Check sheet for the modelled part. Datum: model origin and axes. Units: mm. A direction names the side the tool comes from. Coordinates: 2 decimals unless noted, no trailing zeros. Loops run counter-clockwise (first coordinate to the right, second up) from the corner with the lowest first, then second, coordinate; pieces in that order, holes last.
```python
from build123d import *

# Parameters (mm, degrees)
SKETCH1_W           = 88.9
SKETCH1_H           = 91.44
BOSS_EXTRUDE1_DEPTH = 44.45
SKETCH2_W           = 8.382
SKETCH2_H           = 20.32
CUT_EXTRUDE1_DEPTH  = 25.4
BOSS_EXTRUDE2_DEPTH = 44.45
SKETCH4_R           = 1.6764
CUT_EXTRUDE4_DEPTH  = 22.098
SKETCH5_R           = 2.9464
CUT_EXTRUDE6_DEPTH  = 43.434
SKETCH7_W           = 12.552336234
SKETCH7_H           = 7.366
CUT_EXTRUDE7_DEPTH  = 22.098


with BuildPart() as part:
    # Sketch1 → Boss-Extrude1 (new body)
    with BuildSketch(Plane(origin=(0, 0, 0), x_dir=(1, 0, 0), z_dir=(0, 1, 0))):
        Rectangle(SKETCH1_W, SKETCH1_H)
    extrude(amount=BOSS_EXTRUDE1_DEPTH)

    # Sketch2 → Cut-Extrude1 (cut)
    with BuildSketch(Plane(origin=(0, 44.45, 0), x_dir=(1, 0, 0), z_dir=(0, 1, 0))):
        with Locations((-5.207, -35.56)):
            Rectangle(SKETCH2_W, SKETCH2_H)
        Polygon((-1.016, -45.72), (39.497, -45.72), (39.497, -17.2466), (9.398, -17.2466), (9.398, -10.16), (-1.016, -10.16), (-1.016, -25.4), align=None)
        Polygon((39.497, 17.2466), (39.497, 45.72), (-1.016, 45.72), (-1.016, 25.4), (-1.016, 10.16), (9.398, 10.16), (9.398, 17.2466), align=None)
        with Locations((-5.207, 35.56)):
            Rectangle(SKETCH2_W, SKETCH2_H)
    extrude(amount=-CUT_EXTRUDE1_DEPTH, mode=Mode.SUBTRACT)

    # Sketch3 → Boss-Extrude2 (add)
    with BuildSketch(Plane(origin=(0, 44.45, 0), x_dir=(1, 0, 0), z_dir=(0, 1, 0))):
        Polygon((52.197, -68.58), (52.197, 68.58), (9.398, 68.58), (9.398, 61.214), (39.497, 61.214), (39.497, 45.72), (44.45, 45.72), (44.45, -45.72), (39.497, -45.72), (39.497, -61.214), (9.398, -61.214), (9.398, -68.58), align=None)
    extrude(amount=-BOSS_EXTRUDE2_DEPTH)

    # Sketch4 → Cut-Extrude4 (cut)
    with BuildSketch(Plane.ZY.offset(-9.398)):
        with Locations((-64.77, 29.21)):
            Circle(SKETCH4_R)
        with Locations((-64.77, 38.1)):
            Circle(SKETCH4_R)
        with Locations((-13.6906, 38.1)):
            Circle(SKETCH4_R)
        with Locations((-13.6906, 29.21)):
            Circle(SKETCH4_R)
        with Locations((13.6906, 38.1)):
            Circle(SKETCH4_R)
        with Locations((13.6906, 29.21)):
            Circle(SKETCH4_R)
        with Locations((64.77, 38.1)):
            Circle(SKETCH4_R)
        with Locations((64.77, 29.21)):
            Circle(SKETCH4_R)
    extrude(amount=-CUT_EXTRUDE4_DEPTH, mode=Mode.SUBTRACT)

    # Sketch5 → Cut-Extrude6 (cut)
    with BuildSketch(Plane.ZY.offset(44.45)):
        with Locations((-13.6906, 38.1)):
            Circle(SKETCH5_R)
        with Locations((-13.6906, 29.21)):
            Circle(SKETCH5_R)
        with Locations((13.6906, 38.1)):
            Circle(SKETCH5_R)
        with Locations((13.6906, 29.21)):
            Circle(SKETCH5_R)
    extrude(amount=-CUT_EXTRUDE6_DEPTH, mode=Mode.SUBTRACT)

    # Sketch7 → Cut-Extrude7 (cut)
    with BuildSketch(Plane(origin=(0, 44.45, 0), x_dir=(1, 0, 0), z_dir=(0, 1, 0))):
        with Locations((33.220831883, -64.897)):
            Rectangle(SKETCH7_W, SKETCH7_H)
        with Locations((33.220831883, 64.897)):
            Rectangle(SKETCH7_W, SKETCH7_H)
    extrude(amount=-CUT_EXTRUDE7_DEPTH, mode=Mode.SUBTRACT)


solid = part.part
```
1) Section check A-A on x = 13. Give the number of separate pieces and of enclosed holes in the cut face, plus the area to 3 significant figures.
Answer sheet:
separate pieces: 3
enclosed holes: 8
area: 3,200 mm2
2) Set-up check for faces 5 (the flat face through (-12, 17, 45.72)), 6 (the flat face through (-5, 32, 25.4)), 7 (the flat face through (-9.398, 32, -35)), 8 (the cylindrical face through (20.29, 27.72, 14.46)): record each of +Z, -Z, +X, -X, +Y, -Y from which the full face is reachable in a straight line by a thin tool's end or side.
Answer sheet:
face 5: -X, +Y, -Y
face 6: +Z, +Y
face 7: -Z, +Y
face 8: -X
3) Section check C-C on y = 20.5. Enter the section's corners in (x, z), plus the area to 3 significant figures.
Answer sheet:
outline: (-44.45, -45.72) - (-9.4, -45.72) - (-9.4, -25.4) - (-1.02, -25.4) - (-1.02, -10.16) - (9.4, -10.16) - (9.4, -17.25) - (39.5, -17.25) - (39.5, -61.21) - (9.4, -61.21) - (9.4, -68.58) - (52.2, -68.58) - (52.2, 68.58) - (9.4, 68.58) - (9.4, 61.21) - (39.5, 61.21) - (39.5, 17.25) - (9.4, 17.25) - (9.4, 10.16) - (-1.02, 10.16) - (-1.02, 25.4) - (-9.4, 25.4) - (-9.4, 45.72) - (-44.45, 45.72) - close
area: 7,070 mm2
4) Section check B-B on z = 64.77. Enter the section's corners in (x, y), plus the area to 3 significant figures.
Answer sheet:
outline: (9.4, 0) - (52.2, 0) - (52.2, 44.45) - (39.5, 44.45) - (39.5, 22.35) - (26.94, 22.35) - (26.94, 27.53) - (9.4, 27.53) - close; (9.4, 30.89) - (26.94, 30.89) - (26.94, 36.42) - (9.4, 36.42) - close; (9.4, 39.78) - (26.94, 39.78) - (26.94, 44.45) - (9.4, 44.45) - close
area: 1,510 mm2
5) Mould release check, pull along Y, two halves, no side actions. Record for faces 1 (the flat face through (52.197, 23, 1)), 2 (the flat face through (31.496, 38, -14)), 3 (the flat face through (3, 0, -1)), 4 (the cylindrical face through (-23.037, 38.23, 10.747)): +Y half, -Y half, draft (parallel to the pull), parting line (faces both ways), or undercut.
Answer sheet:
face 1: draft
face 2: undercut
face 3: -Y half
face 4: undercut
6) Depth check by flat-ended pin: pin 1 (2.5 mm diameter, centred on y = 38.1, z = -64.77, fed in from -X); pin 2 (10 mm diameter, centred on x = -18.5, y = 5, fed in from +Z); pin 3 (10 mm diameter, centred on x = -13.5, y = 11.5, fed in from -Z). Enter the tip coordinate at first touch or a pass-through.
Answer sheet:
pin 1: stops at x = 39.5
pin 2: stops at z = 45.72
pin 3: stops at z = -45.72
7) Section check D-D on x = -13. Enter the section's corners in (y, z), plus the area to 3 significant figures.
Answer sheet:
outline: (0, -45.72) - (44.45, -45.72) - (44.45, 45.72) - (0, 45.72) - close; hole circle Ø5.89 at (29.21, -13.69); hole circle Ø5.89 at (29.21, 13.69); hole circle Ø5.89 at (38.1, -13.69); hole circle Ø5.89 at (38.1, 13.69)
area: 3,960 mm2
8) Scan lines: line 1 (Z direction, x = -14, y = 29); line 2 (Y direction, x = 23, z = -64.77); line 3 (Z direction, x = 15.5, y = 41). Record each from-to range of solid material in increasing order.
Answer sheet:
line 1: z = -45.72 to -16.63, -10.75 to 10.75, 16.63 to 45.72
line 2: y = 0 to 27.53, 30.89 to 36.42, 39.78 to 44.45
line 3: z = -68.58 to -61.21, -17.25 to 17.25, 61.21 to 68.58
